Autodesk Inventor part; units mm, degrees
ref_plane "YZ Plane" through (0, 0, 0) normal (1, 0, 0) x (0, 1, 0)
ref_plane "XZ Plane" through (0, 0, 0) normal (0, 1, 0) x (-1, 0, 0)
ref_plane "XY Plane" through (0, 0, 0) normal (0, 0, 1) x (1, 0, 0)
sketch "スケッチ1" plane through (0, 0, 0) normal (0, 0, 1) x (1, 0, 0)
  line L0 (0, 0) -> (110, 0)
  line L1 (110, 0) -> (110, 45)
  line L2 (110, 45) -> (0, 45)
  line L3 (0, 45) -> (0, 0)
  line L4 (0, 32.5) -> (110, 32.5) construction
  line L5 (0, 10) -> (110, 10) construction
  circle A0 centre (10, 10) radius 2.75
  circle A1 centre (100, 10) radius 2.75
  circle A2 centre (30, 32.5) radius 1.75
  circle A3 centre (80, 32.5) radius 1.75
  line L6 (55, 45) -> (55, 0) construction
  dimension "d2" = 110
  dimension "d3" = 45
  dimension "d4" = 12.5
  dimension "d5" = 10
  dimension "d6" = 50
  dimension "d8" = 10
  dimension "d9" = 5.5
  dimension "d10" = 3.5
extrude "押し出し1" add sketch "スケッチ1" along normal blind 20
sketch "スケッチ2" plane through (0, 0, 0) normal (0, 0, -1) x (-1, 0, 0)
  line L0 (0, 0) -> (-110, 0)
  line L1 (-110, 0) -> (0, 0)
  line L2 (0, 0) -> (0, 20)
  line L3 (0, 20) -> (-110, 20)
  line L4 (-110, 20) -> (-110, 0)
  point P0 (-110, 45)
  dimension "d14" = 20
extrude "押し出し2" cut sketch "スケッチ2" against normal blind 12
fillet "フィレット1" radius 2 6 edges at (110, 0, 16) (110, 45, 10) (0, 0, 16) (0, 45, 10) (110, 20, 6) (0, 20, 6)
properties part number "_3D プリント"
Design review of the part built by this model. Coordinates are the model's own, in mm. A direction names the side the tool comes from. Coordinates: 2 decimals unless noted, no trailing zeros. Loops run counter-clockwise (first coordinate to the right, second up) from the corner with the lowest first, then second, coordinate; pieces in that order, holes last. Notation, with made-up numbers: (-4.5, 2) - (28.5, 2) arc R9 cw to (28.5, 13) - close; hole circle Ø10 at (-0.75, -34.5). An arc over 180 degrees is marked (long way). Use CSV: the item, a comma, the result in double quotes. Start each with the question number.
1) Tool access review of faces 4 (the cylindrical face through (0.6, 44.43, 10.14)), 5 (the flat face through (54, 20, 6)), 6 (the cylindrical face through (109.4, 20.57, 6.08)), 7 (the cylindrical face through (0.57, 20.6, 6.08)): name each direction out of +Z, -Z, +X, -X, +Y, -Y from which nothing blocks a thin tool from reaching the whole face with its end or side.
2) For pin 1 Ø10 at (x, z) = (41, 6.5) entering from -Y; pin 2 Ø9 at (x, y) = (10, 10) entering from -Z, all flat-tipped, find the tip position at first contact; note any pin that passes through.
3) The part is to be moulded in two halves that separate along Y. For faces 1 (the cylindrical face through (12.62, 9.17, 15.94)), 2 (the flat face through (0, 27, 12)), 3 (the cylindrical face through (109.4, 0.57, 16.06)), say which applies: +Y half, -Y half, draft (parallel to the pull), parting line (faces both ways), or undercut.
4) Consider section C-C on z = 10.5. Write out the cut boundary in (x, y).
5) Wall thickness on L1, parallel to Y at x = 100, z = 18; L2, parallel to X at y = 32, z = 1.25; L3, parallel to Y at x = 80, z = 15.75: over which ranges is each line inside the solid? List them lowest first. Write a range as from..to.
6) Consider section D-D on x = 42. Write out the cut boundary in (y, z), then the cut area to 3 significant figures.
7) Consider section A-A on y = 10. Write out the cut boundary in (x, z), then the cut area to 3 significant figures.
8) Consider section B-B on x = 30. Write out the cut boundary in (y, z), then the cut area to 3 significant figures.
Geometry says:
1,face 4,"+Z, -Z, -X, +Y"
1,face 5,"-Z, +X, -X, -Y"
1,face 6,"-Z, +X, -Y"
1,face 7,"-Z, -X, -Y"
2,pin 1,"y = 20"
2,pin 2,"z = 12"
3,face 1,"undercut"
3,face 2,"draft"
3,face 3,"-Y half"
4,outline,"(0, 22) arc R2 ccw to (2, 20) - (108, 20) arc R2 ccw to (110, 22) - (110, 43) arc R2 ccw to (108, 45) - (2, 45) arc R2 ccw to (0, 43) - close; hole circle Ø3.5 at (30, 32.5); hole circle Ø3.5 at (80, 32.5)"
5,L1,"0..7.25, 12.75..45"
5,L2,"0..28.32, 31.68..78.32, 81.68..110"
5,L3,"0..30.75, 34.25..45"
6,outline,"(0, 12) - (20, 12) - (20, 0) - (45, 0) - (45, 20) - (0, 20) - close"
6,area,"660 mm^2"
7,outline,"(0, 12) - (7.25, 12) - (7.25, 20) - (0, 20) - close; (12.75, 12) - (97.25, 12) - (97.25, 20) - (12.75, 20) - close; (102.75, 12) - (110, 12) - (110, 20) - (102.75, 20) - close"
7,area,"792 mm^2"
8,outline,"(0, 12) - (20, 12) - (20, 0) - (30.75, 0) - (30.75, 20) - (0, 20) - close; (34.25, 0) - (45, 0) - (45, 20) - (34.25, 20) - close"
8,area,"590 mm^2"
